from build123d import *

# Parameters (mm, degrees)
SLOT_DEPTH      = 75.606467548
SLOT_DEPTH_BACK = 75.606467548
SLOTSKE_W       = 4.69310445
SLOTSKE_H       = 2.101390052
FILLET1_R       = 4


with BuildPart() as part:
    # BodySke → Base-Revolve (revolve)
    with BuildSketch(Plane.XY, mode=Mode.PRIVATE) as base_revolve_sk:
        Polygon((69, 5), (70, 4), (70, 0), (0, 0), (0, 17.45), (0.8, 18.25), (7.2, 18.25), (8, 17.45), (8, 10), (25, 10), (25, 5), align=None)
    revolve(base_revolve_sk.sketch.rotate(Axis((-25.4, 0, 0), (1, 0, 0)), 90), axis=Axis((-25.4, 0, 0), (1, 0, 0)))

    # SlotSke → Slot (cut, two sides: drawn at the far end of the back side and taken through both)
    with BuildSketch(Plane.XY.offset(-SLOT_DEPTH_BACK)):
        Rectangle(SLOTSKE_W, SLOTSKE_H)
    extrude(amount=SLOT_DEPTH + SLOT_DEPTH_BACK, mode=Mode.SUBTRACT)

    # Fillet1
    fillet1_edges = [part.edges().sort_by_distance(p)[0] for p in [
        (8, 0, -10),
    ]]
    fillet(fillet1_edges, radius=FILLET1_R)


solid = part.part
Part model, mm, in its own coordinate system. A direction names the side the tool comes from. Give positions to 0.01 mm unless a question says otherwise; leave off trailing zeros. Loops run counter-clockwise (first coordinate to the right, second up) from the corner with the lowest first, then second, coordinate; pieces in that order, holes last. Notation, with made-up numbers: M -28.5,64.5 L 30.5,64.5 A25 cw 30.5,84.5 Z; hole C 61,82.5 d11. An arc over 180 degrees is marked long. Put each result on its own line as item: value. Start each with the question number.
1) Saw through at A-A (y = 0). List the corners of the cut face in (x, z), then the cut area to 3 significant figures.
2) 3-axis set-ups, long thin cutter, end or side, ignore diameter. For faces 4 (the flat face through (8, -14.3, -0.1)), 5 (the flat face through (1, -1.051, 0)), 6 (the flat face through (70, 0, 0)): which of +Z, -Z, +X, -X, +Y, -Y reach the whole face in a straight line?
3) Flat gauge pins, fed straight in: pin 1 (0.7 mm diameter, centred on x = 1, z = -6, fed in from +Y); pin 2 (0.7 mm diameter, centred on x = 1, z = 1.5, fed in from -Y); pin 3 (5 mm diameter, centred on x = 55, z = -6.5, fed in from -Y); pin 4 (1.5 mm diameter, centred on x = 34, y = -7.5, fed in from +Z). Where does each tip first touch, or does it go through?
4) Saw through at C-C (x = 27). List the corners of the cut face in (y, z).
5) Saw through at B-B (z = 0). List the corners of the cut face in (x, y).
6) Probe probe 1 along Y at (x, z) = (36, 0); probe 2 along X at (y, z) = (0.5, 1); probe 3 along X at (y, z) = (8.5, -4). List the from-to ranges inside material, lowest first.
7) Pull direction Y, two halves, no side cores. Call faces 1 (the cylindrical face through (19, 0, -10)), 2 (the flat face through (2.347, 0, 0)), 3 (the conical face through (0.139, 17.585, -0.373)): +Y half, -Y half, draft (parallel to the pull), parting line (faces both ways), or undercut.
Numbers:
1. outline: M 2.35,-18.25 L 7.2,-18.25 L 8,-17.45 L 8,-14 A4 cw 12,-10 L 25,-10 L 25,-5 L 69,-5 L 70,-4 L 70,4 L 69,5 L 25,5 L 25,10 L 12,10 A4 cw 8,14 L 8,17.45 L 7.2,18.25 L 2.35,18.25 Z
1. area: 1,000 mm^2
2. face 4: +X
2. face 5: +Z, -Z, -X
2. face 6: +Z, -Z, +X, +Y, -Y
3. pin 1: y = 17.35
3. pin 2: y = -18.21
3. pin 3: y = -3
3. pin 4: through
4. outline: C 0,0 d10
5. outline: M 0,-17.45 L 0.8,-18.25 L 7.2,-18.25 L 8,-17.45 L 8,-14 A4 cw 12,-10 L 25,-10 L 25,-5 L 69,-5 L 70,-4 L 70,4 L 69,5 L 25,5 L 25,10 L 12,10 A4 cw 8,14 L 8,17.45 L 7.2,18.25 L 0.8,18.25 L 0,17.45 L 0,1.05 L 2.35,1.05 L 2.35,-1.05 L 0,-1.05 Z
6. probe 1: -5 to 5
6. probe 2: 2.35 to 70
6. probe 3: 0 to 25
7. face 1: parting line
7. face 2: undercut
7. face 3: +Y half
